from build123d import *

# Parameters (mm, degrees)
BOSS_EXTRUDE1_DEPTH     = 1.5875
FILLET1_R               = 3.175
SKETCH2_R               = 4.750027573
SKETCH2_R_2             = 1.830008083
CUT_EXTRUDE1_DEPTH      = 1
CUT_EXTRUDE1_DEPTH_BACK = 2.5875
SKETCH3_R               = 0.635
CUT_EXTRUDE2_DEPTH      = 1
CUT_EXTRUDE2_DEPTH_BACK = 2.5875


with BuildPart() as part:
    # Sketch1 → Boss-Extrude1 (new body)
    with BuildSketch(Plane(origin=(0, 0, 0), x_dir=(1, 0, 0), z_dir=(0, 1, 0))):
        with BuildLine():
            Line((-8.89, -66.675), (-43.815, -66.675))
            Line((-43.815, -66.675), (-43.815, -1.27))
            ThreePointArc((-43.815, -1.27), (-43.443025612, -0.371974388), (-42.545, 0))
            Line((-42.545, 0), (42.545, 0))
            Line((42.545, 0), (42.545, -54.843091388))
            Line((42.545, -54.843091388), (-2.54, -54.843091388))
            Line((-2.54, -54.843091388), (-2.54, -73.025))
            ThreePointArc((-2.54, -73.025), (-4.399871939, -68.534871939), (-8.89, -66.675))
        make_face()
    extrude(amount=BOSS_EXTRUDE1_DEPTH)

    # Fillet1
    fillet1_edges = [part.edges().sort_by_distance(p)[0] for p in [
        (-2.54, 0.79375, 54.843091388),
    ]]
    fillet(fillet1_edges, radius=FILLET1_R)

    # Sketch2 → Cut-Extrude1 (cut, two sides)
    with BuildSketch(Plane(origin=(0, 1.5875, 0), x_dir=(-1, 0, 0), z_dir=(0, 1, 0))) as cut_extrude1_sk:
        with Locations((26.115028378, 39.200331632)):
            Circle(SKETCH2_R)
        with Locations((24.115016768, 53.700415803)):
            Circle(SKETCH2_R_2)
        with Locations((24.114889767, 12.7)):
            Circle(SKETCH2_R_2)
    extrude(amount=CUT_EXTRUDE1_DEPTH, mode=Mode.SUBTRACT)
    extrude(cut_extrude1_sk.sketch, amount=-CUT_EXTRUDE1_DEPTH_BACK, mode=Mode.SUBTRACT)

    # Sketch3 → Cut-Extrude2 (cut, two sides)
    with BuildSketch(Plane(origin=(0, 1.5875, 0), x_dir=(-1, 0, 0), z_dir=(0, 1, 0))) as cut_extrude2_sk:
        with Locations((27.305, 3.175)):
            Circle(SKETCH3_R)
        with Locations((13.97, 3.175)):
            Circle(SKETCH3_R)
        with Locations((0.635, 3.175)):
            Circle(SKETCH3_R)
        with Locations((-12.7, 3.175)):
            Circle(SKETCH3_R)
        with Locations((-26.035, 3.175)):
            Circle(SKETCH3_R)
        with Locations((-39.37, 3.175)):
            Circle(SKETCH3_R)
        with Locations((-39.37, 15.298272847)):
            Circle(SKETCH3_R)
        with Locations((-39.37, 27.421545694)):
            Circle(SKETCH3_R)
        with Locations((-39.37, 39.544818541)):
            Circle(SKETCH3_R)
        with Locations((-39.37, 51.668091388)):
            Circle(SKETCH3_R)
        with Locations((-28.09875, 51.668091388)):
            Circle(SKETCH3_R)
        with Locations((-16.8275, 51.668091388)):
            Circle(SKETCH3_R)
        with Locations((-5.55625, 51.668091388)):
            Circle(SKETCH3_R)
        with Locations((5.715, 51.668091388)):
            Circle(SKETCH3_R)
        with Locations((5.715, 63.5)):
            Circle(SKETCH3_R)
        with Locations((17.356666667, 63.5)):
            Circle(SKETCH3_R)
        with Locations((28.998333333, 63.5)):
            Circle(SKETCH3_R)
        with Locations((40.64, 63.5)):
            Circle(SKETCH3_R)
        with Locations((40.64, 51.435)):
            Circle(SKETCH3_R)
        with Locations((40.64, 39.37)):
            Circle(SKETCH3_R)
        with Locations((40.64, 27.305)):
            Circle(SKETCH3_R)
        with Locations((40.64, 15.24)):
            Circle(SKETCH3_R)
        with Locations((40.64, 3.175)):
            Circle(SKETCH3_R)
    extrude(amount=CUT_EXTRUDE2_DEPTH, mode=Mode.SUBTRACT)
    extrude(cut_extrude2_sk.sketch, amount=-CUT_EXTRUDE2_DEPTH_BACK, mode=Mode.SUBTRACT)


solid = part.part
Work out the finished part from the listing and answer in its coordinate system (mm). Give positions to 0.01 mm unless a question says otherwise; leave off trailing zeros. Order: outer loops, then holes, each group sorted by start corner. A loop starts at its lowest first (then second) coordinate and runs counter-clockwise, first axis right, second up. Notation, with made-up numbers: (-26, 75.5) -> (-7, 75.5) arc R17 ccw to (-7, 95.5) -> close; hole circle Ø1 at (79, 70). An arc over 180 degrees is marked (long way). Answer as a JSON object with one key per item and string values. Group by question number.
1. A flat-ended cylindrical pin translates along its axis: pin 1 Ø1.7 at (x, z) = (-40.64, 63.5) entering from -Y. Find the tip coordinate at first contact, or state that the pin passes through.
2. Section C-C on z = 43 is taken. Determine the outline of the cut face in (x, y) (1 decimal).
3. The mould has two halves that part along Z. Classify faces 1 (the cylindrical face through (-22.77, 0.8, 13.94)), 2 (the cylindrical face through (-23.718, 0.805, 51.914)), 3 (the flat face through (0, 0, 28)), 4 (the cylindrical face through (-4.351, 0.783, 68.585)): released by +Z, released by -Z, zero draft, split by the parting line, or undercut.
4. Section B-B on x = -36.5 is taken. Determine the outline of the cut face in (y, z) (1 decimal), plus the area to 3 significant figures.
5. Consider line 1 along X through (y, z) = (0.8, 63.5) (3 decimals); line 2 along Z through (x, y) = (-13.97, 0.85) (3 decimals); line 3 along X through (y, z) = (0.2, 15.5) (3 decimals). Determine where each line is inside the solid, lowest interval first. Write a range as [from, to].
6. Section D-D on y = 0.9 is taken. Count the separate pieces of the cut face and the enclosed holes in it, plus the area to 3 significant figures.
7. Section A-A on z = 12.7 is taken. Determine the outline of the cut face in (x, y) (1 decimal), plus the area to 3 significant figures.
Result sheet:
{
 "1": {"pin 1": "stops at y = 0"},
 "2": {"outline": "(-43.8, 0) -> (-29, 0) -> (-29, 1.6) -> (-43.8, 1.6) -> close; (-23.3, 0) -> (42.5, 0) -> (42.5, 1.6) -> (-23.3, 1.6) -> close"},
 "3": {"face 1": "undercut", "face 2": "undercut", "face 3": "zero draft", "face 4": "released by +Z"},
 "4": {"outline": "(0, 0) -> (1.6, 0) -> (1.6, 66.7) -> (0, 66.7) -> close", "area": "106 mm^2"},
 "5": {"line 1": "x = [-43.815, -41.275], [-40.005, -29.633], [-28.363, -17.992], [-16.722, -6.35], [-5.08, -2.54]", "line 2": "z = [0, 2.54], [3.81, 66.675]", "line 3": "x = [-43.815, -41.219], [-40.061, 38.768], [39.972, 42.545]"},
 "6": {"separate pieces": "1", "enclosed holes": "26", "area": "5,110 mm^2"},
 "7": {"outline": "(-43.8, 0) -> (-25.9, 0) -> (-25.9, 1.6) -> (-43.8, 1.6) -> close; (-22.3, 0) -> (42.5, 0) -> (42.5, 1.6) -> (-22.3, 1.6) -> close", "area": "131 mm^2"}
}
